Geometry check sheet. Reference: the model listing, model coordinates, mm. A direction names the side the tool comes from. Round coordinates to 2 decimals unless told otherwise and drop trailing zeros. Loops run counter-clockwise (first coordinate to the right, second up) from the corner with the lowest first, then second, coordinate; pieces in that order, holes last.
Autodesk Inventor part; units mm, degrees
ref_plane "YZ Plane" through (0, 0, 0) normal (1, 0, 0) x (0, 1, 0)
ref_plane "XZ Plane" through (0, 0, 0) normal (0, 1, 0) x (-1, 0, 0)
ref_plane "XY Plane" through (0, 0, 0) normal (0, 0, 1) x (1, 0, 0)
sketch "Sketch1" plane through (0, 0, 0) normal (0, 0, 1) x (1, 0, 0)
  line L0 (-39, 53) -> (6, 53)
  line L1 (6, 53) -> (6, 44)
  line L2 (6, 44) -> (-39, 44)
  line L3 (-39, 44) -> (-39, 53)
  line L4 (0, 44) -> (6, 44)
  line L5 (6, 44) -> (6, 0)
  line L6 (6, 0) -> (0, 0)
  line L7 (0, 0) -> (0, 44)
  line L8 (6, 53) -> (45, 53)
  line L9 (45, 53) -> (45, 44)
  line L10 (45, 44) -> (6, 44)
  line L11 (6, 44) -> (6, 53)
  dimension "d1" = 9
  dimension "d2" = 45
  dimension "d3" = 6
  dimension "d17" = 53
  dimension "d19" = 45
extrude "Extrusion1" add sketch "Sketch1" along normal blind 3
fillet "Fillet1" radius 15 2 edges at (0, 44, 1.5) (6, 44, 1.5)
sketch "Sketch2" plane through (0, 0, 3) normal (0, 0, 1) x (1, 0, 0)
  line L0 (45, 53) -> (-39, 53)
  line L1 (6, 0) -> (6, 29)
  point P0 (0, 0)
  point P1 (3, 44)
  point P2 (6, 44)
  point P3 (-15, 44)
  dimension "d20" = 3
hole "Hole1" at (3, 44, 3) direction (0, 0, -1) diameter 6 end through all
sketch "Sketch3" plane through (0, 0, 3) normal (0, 0, 1) x (1, 0, 0)
  line L0 (-39, 53) -> (-39, 44)
  line L1 (45, 53) -> (-39, 53)
  line L2 (45, 44) -> (45, 53)
  point P0 (0, 0)
  point P1 (-31.5, 50)
  point P2 (-39, 48.5)
  dimension "d29" = 3
  dimension "d31" = 7.5
hole "Hole2" at (-31.5, 50, 3) direction (0, 0, -1) diameter 3.4 end through all
equation "\"d19\" = d2"
properties part number "Top_Separator Lever" material "Nylon 6/6"
1) Sectioned sample at D-D, the plane y = 24.5. Record the cut outline in (x, z), then the cut area to 3 significant figures.
Report:
outline: (0, 0) - (6, 0) - (6, 3) - (0, 3) - close
area: 18.0 mm2
2) Scan lines: line 1 along Y through (x, z) = (-31.5, 2.15); line 2 along Y through (x, z) = (3, 1.25); line 3 along X through (y, z) = (50, 2.25). Record each from-to range of solid material in increasing order.
Report:
line 1: y = 44 to 48.3, 51.7 to 53
line 2: y = 0 to 41, 47 to 53
line 3: x = -39 to -33.2, -29.8 to 45
3) Sectioned sample at C-C, the plane z = 1.15. Record the cut outline in (x, y).
Report:
outline: (-39, 44) - (-15, 44) arc R15 cw to (0, 29) - (0, 0) - (6, 0) - (6, 29) arc R15 cw to (21, 44) - (45, 44) - (45, 53) - (-39, 53) - close; hole circle Ø3.4 at (-31.5, 50); hole circle Ø6 at (3, 44)
4) Sectioned sample at A-A, the plane x = 3. Record the cut outline in (y, z).
Report:
outline: (0, 0) - (41, 0) - (41, 3) - (0, 3) - close; (47, 0) - (53, 0) - (53, 3) - (47, 3) - close
5) Sectioned sample at B-B, the plane y = 50. Record the cut outline in (x, z).
Report:
outline: (-39, 0) - (-33.2, 0) - (-33.2, 3) - (-39, 3) - close; (-29.8, 0) - (45, 0) - (45, 3) - (-29.8, 3) - close
6) Access from +Z, -Z, +X, -X, +Y, -Y to the whole of each face (thin tool, end or side, straight path). Record for faces 4 (the face through (6, 15, 1)), 5 (the face through (-27, 44, 1)), 6 (the face through (3, 0, 1)).
Report:
face 4: +Z, -Z, +X, -Y
face 5: +Z, -Z, -X, -Y
face 6: +Z, -Z, +X, -X, -Y
7) Mould release check, pull along Y, two halves, no side actions. Record for faces 1 (the face through (0, 14, 1)), 2 (the face through (2, 53, 1)), 3 (the face through (3, 47, 1)): +Y half, -Y half, draft (parallel to the pull), parting line (faces both ways), or undercut.
Report:
face 1: draft
face 2: +Y half
face 3: undercut
8) Gauge pin test, flat ends, axial feed: pin 1 (1.5 mm diameter, centred on y = 9, z = 1, fed in from -X); pin 2 (5.5 mm diameter, centred on x = 3, y = 44, fed in from -Z); pin 3 (1.5 mm diameter, centred on x = 27, z = 2, fed in from -Y); pin 4 (1.5 mm diameter, centred on y = 42, z = 2.5, fed in from +X). Record the tip position at first contact, or that the pin passes through.
Report:
pin 1: stops at x = 0
pin 2: passes through
pin 3: stops at y = 44
pin 4: stops at x = 15.01
